from build123d import *

# Parameters (mm, degrees)
SKETCH1_W                = 500
SKETCH1_H                = 50
BOSS_EXTRUDE1_DEPTH      = 10
CUT_EXTRUDE1_DEPTH       = 11
BOSS_EXTRUDE3_DEPTH      = 2
BOSS_EXTRUDE3_DEPTH_BACK = 12
SKETCH4_W                = 115.032991515
SKETCH4_H                = 5
CUT_EXTRUDE2_DEPTH       = 5


with BuildPart() as part:
    # Sketch1 → Boss-Extrude1 (new body)
    with BuildSketch(Plane.XY):
        with Locations((283.352405613, 0)):
            Rectangle(SKETCH1_W, SKETCH1_H)
    extrude(amount=BOSS_EXTRUDE1_DEPTH)

    # Sketch2 → Cut-Extrude1 (cut, through all)
    with BuildSketch(Plane.XY.offset(10)):
        Polygon((533.352405613, 0), (85.627765445, -25), (533.352405613, -25), align=None)
        with BuildLine():
            Line((33.352405613, -25), (81.993040664, -25))
            ThreePointArc((81.993040664, -25), (56.907700084, -19.408398641), (35.752423976, -4.814063764))
            ThreePointArc((35.752423976, -4.814063764), (33.571532765, 2.680644565), (38.404725068, 8.809852636))
            ThreePointArc((38.404725068, 8.809852636), (66.634144242, 19.90850289), (96.536599016, 25))
            Line((96.536599016, 25), (33.352405613, 25))
            Line((33.352405613, 25), (33.352405613, -25))
        make_face()
        Polygon((115.905115224, 25), (533.352405613, 15), (533.352405613, 25), align=None)
    extrude(amount=-CUT_EXTRUDE1_DEPTH, mode=Mode.SUBTRACT)

    # Sketch3 → Boss-Extrude3 (add, two sides)
    with BuildSketch(Plane(origin=(0, 0, 0), x_dir=(-1, 0, 0), z_dir=(0, 0, -1))) as boss_extrude3_sk:
        Polygon((-159.0031787, 23.967580711), (-274.0031787, 21.212741893), (-274.0031787, 17.212741893), (-159.0031787, 19.967580711), align=None)
    extrude(amount=BOSS_EXTRUDE3_DEPTH)
    extrude(boss_extrude3_sk.sketch, amount=-BOSS_EXTRUDE3_DEPTH_BACK)

    # Sketch4 → Cut-Extrude2 (cut)
    with BuildSketch(Plane(origin=(0.665008284, 27.760590609, 0), x_dir=(0.9997132, -0.02394825, 0), z_dir=(0.02394825, 0.9997132, 0))):
        with Locations((215.900090662, -5)):
            Rectangle(SKETCH4_W, SKETCH4_H)
    extrude(amount=-CUT_EXTRUDE2_DEPTH, mode=Mode.SUBTRACT)


solid = part.part
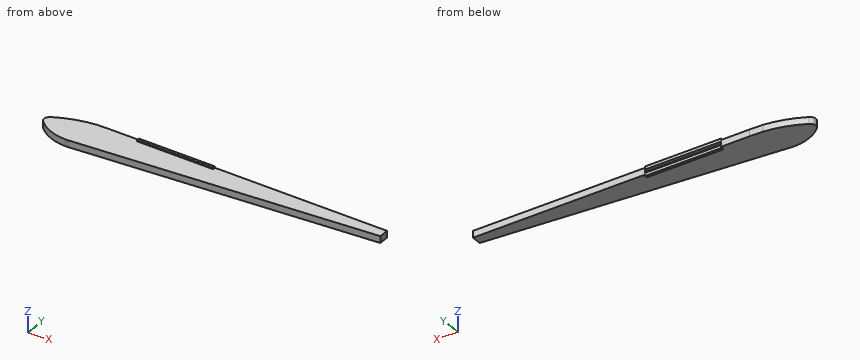
Design review of the part built by this model. Coordinates are the model's own, in mm. Round coordinates to 2 decimals unless told otherwise and drop trailing zeros. Write each loop counter-clockwise with the first axis right and the second up, starting at its lowest first coordinate (ties: lowest second). Pieces come first, ordered by that corner, then holes. Notation, with made-up numbers: M -37,73 L 8,73 A14 ccw 8,77 Z; hole C 12,29.5 d2. An arc over 180 degrees is marked long. One line per item, written item: value. Start each with the question number.
1. Clearance check with flat-ended pins moving along their axes: P1, Ø2, axis at x = 386.5, z = 7, coming from the -Y side; P2, Ø12, axis at x = 280.5, y = -15.5, coming from the +Z side; P3, Ø8, axis at x = 394.5, z = 10.5, coming from the -Y side. State where each tip first meets the part, or that it passes through.
2. Take a section at B-B on y = 4.5. State the section outline as (x, z) points.
3. To check wall thickness, follow probe 1 along Z at (x, y) = (314, -1); probe 2 along Y at (x, z) = (192.5, 10.75); probe 3 along Y at (x, z) = (173, 5.75). State the ranges of each line that lie inside material, in increasing order. Write a range as from..to.
4. Take a section at C-C on x = 413. State the section outline as (y, z) points, then the cut area to 3 significant figures.
5. Take a section at A-A on x = 257. State the section outline as (y, z) points.
Computed:
1. P1: stops at y = -8.26
1. P2: stops at z = 10
1. P3: stops at y = -7.97
2. outline: M 34.14,0 L 533.35,0 L 533.35,10 L 34.14,10 Z
3. probe 1: z = 0..10
3. probe 2: y = 19.17..23.17
3. probe 3: y = -20.12..18.63
4. outline: M -6.72,0 L 17.88,0 L 17.88,10 L -6.72,10 Z
4. area: 246 mm²
5. outline: M -15.43,0 L 17.62,0 L 17.62,-2 L 21.62,-2 L 21.62,2.5 L 16.62,2.5 L 16.62,7.5 L 21.62,7.5 L 21.62,12 L 17.62,12 L 17.62,10 L -15.43,10 Z
